Study the drawing (mm; zero at the part's minimum x, y, z) and answer. Coordinates: 2 decimals unless noted, no trailing zeros. Loops run counter-clockwise (first coordinate to the right, second up) from the corner with the lowest first, then second, coordinate; pieces in that order, holes last. Notation, with made-up numbers: (22, 52) -> (44, 52) arc R18 ccw to (44, 87) -> close; hole circle Ø2 at (-23.5, 7). An arc over 180 degrees is marked (long way). Answer in a Markdown table with one row per item.
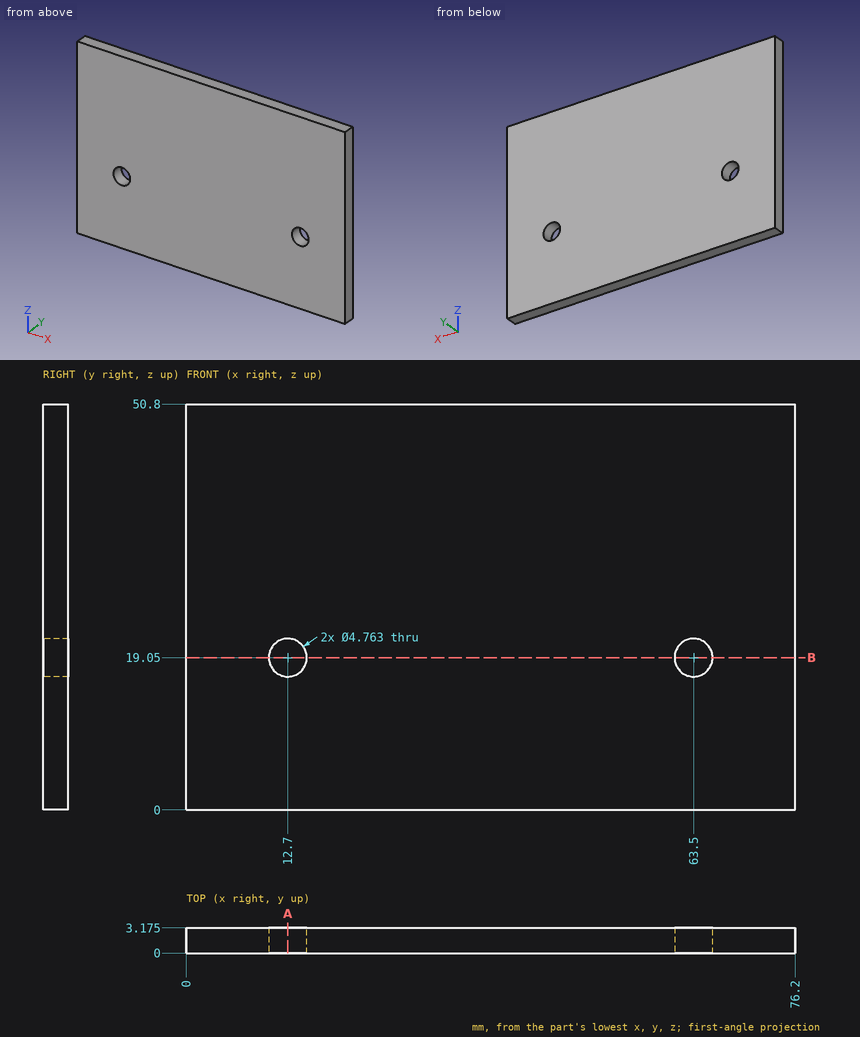
1. Given pin 1 Ø6 at (x, z) = (25.5, 25.5) entering from -Y; pin 2 Ø4.5 at (x, z) = (63.5, 19.05) entering from +Y, each flat-ended and moving along its own axis, determine where each tip first touches the part or whether it passes through.
A:
| item | result |
|---|---|
| pin 1 | stops at y = 0 |
| pin 2 | passes through |
2. A cutting plane is placed at A-A on x = 12.7. Give the vertices of the cut face in (y, z) (1 decimal), and give its area (3 significant figures).
A:
| item | result |
|---|---|
| outline | (0, 0) -> (3.2, 0) -> (3.2, 16.7) -> (0, 16.7) -> close; (0, 21.4) -> (3.2, 21.4) -> (3.2, 50.8) -> (0, 50.8) -> close |
| area | 146 mm2 |
3. Find the intervals of material crossed by probe 1 along Z at (x, y) = (12.7, 1.65), in increasing order.
A:
| item | result |
|---|---|
| probe 1 | z = 0 to 16.67, 21.43 to 50.8 |
4. A cutting plane is placed at B-B on z = 19.05. Give the vertices of the cut face in (x, y) (1 decimal).
A:
| item | result |
|---|---|
| outline | (0, 0) -> (10.3, 0) -> (10.3, 3.2) -> (0, 3.2) -> close; (15.1, 0) -> (61.1, 0) -> (61.1, 3.2) -> (15.1, 3.2) -> close; (65.9, 0) -> (76.2, 0) -> (76.2, 3.2) -> (65.9, 3.2) -> close |
